```python
from build123d import *

# Parameters (mm, degrees)
LINEAR_AUSTRAGEN1_DEPTH = 1


with BuildPart() as part:
    # Außenkontur → Linear austragen1 (new body, symmetric)
    with BuildSketch(Plane.XY):
        with BuildLine():
            Line((-83, 0), (-57, 0))
            ThreePointArc((-57, 0), (-52, 5), (-47, 0))
            Line((-47, 0), (-44, 0))
            ThreePointArc((-44, 0), (-44.254033308, 2), (-45, 3.872983346))
            ThreePointArc((-45, 3.872983346), (-46.916580756, 42.566918881), (-17.5, 67.777208559))
            ThreePointArc((-17.5, 67.777208559), (-8.441984355, 64.845892989), (-7.240867658, 55.401446097))
            ThreePointArc((-7.240867658, 55.401446097), (-6.75320549, 47.711152181), (0, 44))
            Line((0, 44), (0, 47))
            ThreePointArc((0, 47), (-5, 52), (0, 57))
            Line((0, 57), (0, 83))
            ThreePointArc((0, 83), (-8.493750568, 81.512894362), (-15.977012787, 77.228496103))
            ThreePointArc((-15.977012787, 77.228496103), (-33.644463337, 65.816474944), (-53.515303741, 58.922801215))
            ThreePointArc((-53.515303741, 58.922801215), (-55.306825995, 58.089224466), (-56.568542495, 56.568542495))
            ThreePointArc((-56.568542495, 56.568542495), (-62.483030705, 42.514608), (-66.293095094, 27.75054166))
            ThreePointArc((-66.293095094, 27.75054166), (-67.776085308, 24.196284331), (-70.608999234, 21.587337453))
            ThreePointArc((-70.608999234, 21.587337453), (-79.682077632, 12.445381054), (-83, 0))
        make_face()
    extrude(amount=LINEAR_AUSTRAGEN1_DEPTH, both=True)


solid = part.part
```
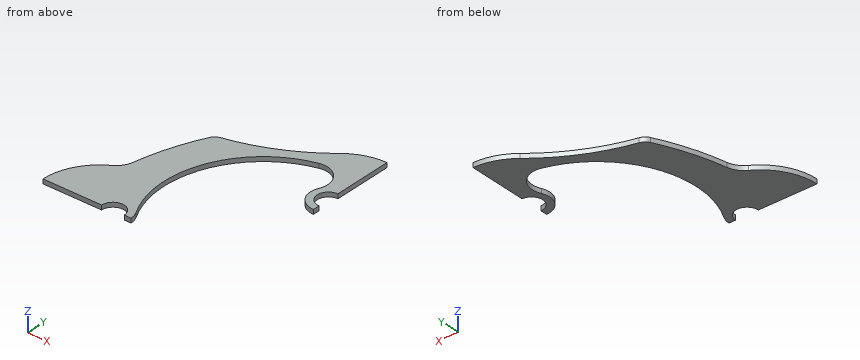
Build history of the part. All positions in model axes, mm. Round coordinates to 2 decimals unless told otherwise and drop trailing zeros. Loops run counter-clockwise (first coordinate to the right, second up) from the corner with the lowest first, then second, coordinate; pieces in that order, holes last.
Item 1: Pin check, flat tip, straight feed: P1, Ø1, axis at y = 70, z = 0, coming from the -X side. Stop position of the tip, or through.
Item 2: Drill centre lines: line 1 along X through (y, z) = (4, 0.2); line 2 along X through (y, z) = (56, -0.3); line 3 along Y through (x, z) = (-32, 0.35). Where is each one in solid material? Low to high.
Item 3: Saw through at C-C (x = -24.5). List the corners of the cut face in (y, z).
Item 4: Saw through at A-A (y = 49.5). List the corners of the cut face in (x, z), then the cut area to 3 significant figures.
Item 5: Saw through at B-B (z = 0.7). List the corners of the cut face in (x, y).
Item 6: Saw through at D-D (x = -52). List the corners of the cut face in (y, z).
Worked answers:
1. P1: stops at x = -26.86
2. line 1: x = -82.68 to -55, -49 to -45.07
2. line 2: x = -56.86 to -37.9, -6.99 to -3
2. line 3: y = 61.03 to 66.64
3. outline: (65.32, -1) - (70.97, -1) - (70.97, 1) - (65.32, 1) - close
4. outline: (-59.84, -1) - (-43.16, -1) - (-43.16, 1) - (-59.84, 1) - close; (-7.6, -1) - (-4.33, -1) - (-4.33, 1) - (-7.6, 1) - close
4. area: 39.9 mm2
5. outline: (-83, 0) - (-57, 0) arc R5 cw to (-47, 0) - (-44, 0) arc R8 ccw to (-45, 3.87) arc R44 cw to (-17.5, 67.78) arc R8.88 cw to (-7.24, 55.4) arc R8 ccw to (0, 44) - (0, 47) arc R5 cw to (0, 57) - (0, 83) arc R25 ccw to (-15.98, 77.23) arc R88 cw to (-53.52, 58.92) arc R4.5 ccw to (-56.57, 56.57) arc R104.68 ccw to (-66.29, 27.75) arc R9 cw to (-70.61, 21.59) arc R25 ccw to start
6. outline: (5, -1) - (59.27, -1) - (59.27, 1) - (5, 1) - close
